Source: CAD feature listing. Evaluate the final solid. Frame: model axes, mm. Give positions to 0.01 mm unless a question says otherwise; leave off trailing zeros. Order: outer loops, then holes, each group sorted by start corner. A loop starts at its lowest first (then second) coordinate and runs counter-clockwise, first axis right, second up. Notation, with made-up numbers: (26, 30) -> (83, 30) arc R32 cw to (83, 65) -> close; hole circle Ø7 at (28.5, 34.25). An arc over 180 degrees is marked (long way). Use CSV: the item, a comma, the result in double quotes.
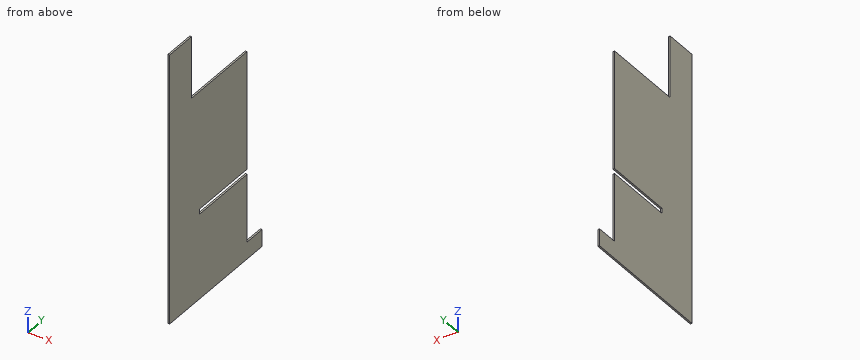
```python
from build123d import *

# Parameters (mm, degrees)
F1_DEPTH = 6


with BuildPart() as f1:
    # F0 (on Right) → F1 (new body)
    with BuildSketch(Plane.YZ):
        Polygon((-368, 218), (-482, 218), (-482, -734), (0, -734), (0, -674), (-60, -674), (-78, -674), (-78, -434), (-326, -434), (-326, -416), (-78, -416), (-78, 0), (-368, 0), align=None)
    extrude(amount=F1_DEPTH)


solid = f1.part
```
1. Section query D-D on y = -339.5. Return loops of the section in (x, z), plus the area to 3 significant figures.
Answer below:
outline,"(0, -734) -> (6, -734) -> (6, 0) -> (0, 0) -> close"
area,"4,400 mm²"
2. Section query B-B on x = 5. Return loops of the section in (y, z), plus the area to 3 significant figures.
Answer below:
outline,"(-482, -734) -> (0, -734) -> (0, -674) -> (-78, -674) -> (-78, -434) -> (-326, -434) -> (-326, -416) -> (-78, -416) -> (-78, 0) -> (-368, 0) -> (-368, 218) -> (-482, 218) -> close"
area,"322,000 mm²"
3. Section query A-A on y = -255. Return loops of the section in (x, z), plus the area to 3 significant figures.
Answer below:
outline,"(0, -734) -> (6, -734) -> (6, -434) -> (0, -434) -> close; (0, -416) -> (6, -416) -> (6, 0) -> (0, 0) -> close"
area,"4,300 mm²"
4. Pin query (flat end, axial travel): P1, Ø3, axis at x = 3.5, y = -217.5, coming from the +Z side; P2, Ø1.8, axis at x = 4.5, y = -35.5, coming from the +Z side; P3, Ø1.8, axis at x = 2, z = 84, coming from the +Y side; P4, Ø12, axis at y = -387, z = 3, coming from the -X side. Return the tip coordinate at first contact, or that it passes through.
Answer below:
P1,"stops at z = 0"
P2,"stops at z = -674"
P3,"stops at y = -368"
P4,"stops at x = 0"
5. Ray query, line 1 along Z through (x, y) = (4.5, -273); line 2 along Y through (x, z) = (2.45, -117); line 3 along Z through (x, y) = (0.4, -349.5). Return the intervals inside material, ascending.
Answer below:
line 1,"z = -734 to -434, -416 to 0"
line 2,"y = -482 to -78"
line 3,"z = -734 to 0"
6. Section query C-C on z = -595. Return loops of the section in (x, y), plus the area to 3 significant figures.
Answer below:
outline,"(0, -482) -> (6, -482) -> (6, -78) -> (0, -78) -> close"
area,"2,420 mm²"
